Work out the finished part from the listing and answer in its coordinate system (mm). Give positions to 0.01 mm unless a question says otherwise; leave off trailing zeros. Write each loop counter-clockwise with the first axis right and the second up, starting at its lowest first coordinate (ties: lowest second). Pieces come first, ordered by that corner, then holes.
1) Straight lines are drawn through the part: probe 1 along Y at (x, z) = (6.5, -2.5); probe 2 along Y at (x, z) = (0.75, 0.5); probe 3 along X at (y, z) = (8.75, -4.75). For each, find the intervals that lie inside material, in ascending order.
2) Find section C-C (z = 4.5). Determine the outline of the cut face in (x, y).
3) Find section A-A (x = 0). Determine the outline of the cut face in (y, z), plus the area to 3 significant figures.
4) Given pin 1 Ø2 at (x, z) = (-10, -1) entering from +Y; pin 2 Ø2 at (y, z) = (4, 0.5) entering from +X; pin 3 Ø4 at (y, z) = (-7.5, -4) entering from +X, each flat-ended and moving along its own axis, determine where each tip first touches the part or whether it passes through.
5) Find section D-D (x = -12). Determine the outline of the cut face in (y, z).
6) Determine the mould class of faces 1 (the face through (10, 3.2, 0.4)), 2 (the face through (5.1, 9.4, 7)), 3 (the face through (12.932, -5.362, 0.409)) for opening direction X: pulls with the +X half, pulls with the -X half, needs draft (parallel to the pull), parting line crosses it, or undercut.
```python
from build123d import *

# Parameters (mm, degrees)
CYLINDER014_R     = 10.5
CYLINDER014_DEPTH = 13
CYLINDER013_R     = 14
CYLINDER013_DEPTH = 13


with BuildPart() as cylinder014:
    # Cylinder014 → Cylinder014 (new body)
    with BuildSketch(Plane.XY.offset(-6)):
        Circle(CYLINDER014_R)
    extrude(amount=CYLINDER014_DEPTH)


with BuildPart() as cut086:
    # Cylinder013 → Cylinder013 (new body)
    with BuildSketch(Plane.XY.offset(-6)):
        Circle(CYLINDER013_R)
    extrude(amount=CYLINDER013_DEPTH)

    # Cut086: cut Cylinder014
    add(cylinder014.part, mode=Mode.SUBTRACT)


solid = cut086.part
```
Results:
1. probe 1: y = -12.4 to -8.25, 8.25 to 12.4
1. probe 2: y = -13.98 to -10.47, 10.47 to 13.98
1. probe 3: x = -10.93 to -5.8, 5.8 to 10.93
2. outline: circle Ø28 at (0, 0); hole circle Ø21 at (0, 0)
3. outline: (-14, -6) - (-10.5, -6) - (-10.5, 7) - (-14, 7) - close; (10.5, -6) - (14, -6) - (14, 7) - (10.5, 7) - close
3. area: 91.0 mm2
4. pin 1: stops at y = 10.72
4. pin 2: stops at x = 13.67
4. pin 3: stops at x = 12.87
5. outline: (-7.21, -6) - (7.21, -6) - (7.21, 7) - (-7.21, 7) - close
6. face 1: undercut
6. face 2: needs draft
6. face 3: parting line crosses it
